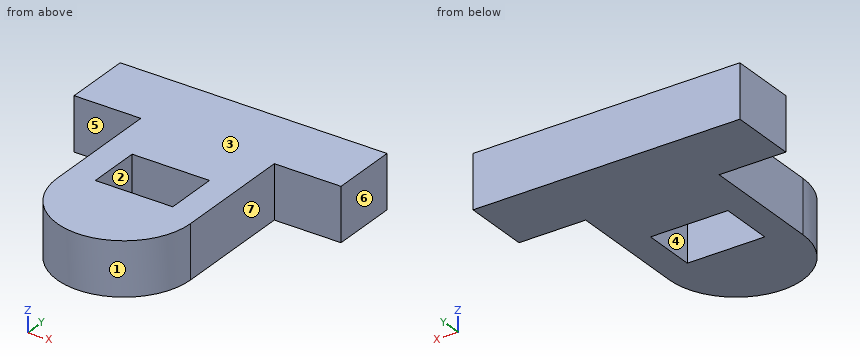
from build123d import *

# Parameters (mm, degrees)
BOSS_EXTRUDE1_DEPTH = 5.08
CUT_EXTRUDE1_DEPTH  = 32.75406374


with BuildPart() as part:
    # Sketch1 → Boss-Extrude1 (new body)
    with BuildSketch(Plane.XY):
        with BuildLine():
            Line((12.7, 18.542), (19.05, 18.542))
            Line((19.05, 18.542), (19.05, 24.892))
            Line((19.05, 24.892), (-6.35, 24.892))
            Line((-6.35, 24.892), (-6.35, 18.542))
            Line((-6.35, 18.542), (0, 18.542))
            Line((0, 18.542), (0, 6.985))
            ThreePointArc((0, 6.985), (6.35, 0.635), (12.7, 6.985))
            Line((12.7, 6.985), (12.7, 18.542))
        make_face()
    extrude(amount=BOSS_EXTRUDE1_DEPTH)

    # Sketch2 → Cut-Extrude1 (cut, through all)
    with BuildSketch(Plane.XY.offset(5.08)):
        Polygon((6.35, 13.462), (10.033, 13.462), (10.033, 8.382), (2.667, 8.382), (2.667, 13.462), align=None)
    extrude(amount=-CUT_EXTRUDE1_DEPTH, mode=Mode.SUBTRACT)


solid = part.part
Geometry: final body of the model. Coordinates: model frame, mm. Face numbers are marked on the shaded views. A direction names the side the tool comes from. Coordinates: 2 decimals unless noted, no trailing zeros. Order: outer loops, then holes, each group sorted by start corner. A loop starts at its lowest first (then second) coordinate and runs counter-clockwise, first axis right, second up. Notation, with made-up numbers: M -18,20 L -4,20 A24 ccw -4,38 Z; hole C -23.75,-29 d2. An arc over 180 degrees is marked long. One line per question, with ' | ' between items. Start each with the question number.
Item 1: Cut plane A-A, the plane x = 6.35. Return the cut outline in (y, z) (3 decimals).
Item 2: Cut plane D-D, the plane y = 16.75. Return the cut outline in (x, z), then the cut area to 3 significant figures.
Item 3: Ray query, probe 1 along X at (y, z) = (12, 4.8); probe 2 along X at (y, z) = (8, 0.3); probe 3 along Y at (x, z) = (15.25, 0.5). Return the intervals inside material, ascending. Write a range as [from, to].
Item 4: Draft query along Y for the marked faces 1, 2 and 3. Return one class per face: released by +Y, released by -Y, zero draft, split by the parting line, or undercut.
Item 5: Pin query (flat end, axial travel): pin 1 Ø2.5 at (y, z) = (12, 1.5) entering from +X; pin 2 Ø2.5 at (x, z) = (16.5, 3.5) entering from -Y; pin 3 Ø1.5 at (x, z) = (8.5, 1) entering from -Y. Return the tip coordinate at first contact, or that it passes through.
Item 6: Cut plane B-B, the plane z = 2. Return the cut outline in (x, y) (3 decimals).
Item 7: Cut plane C-C, the plane x = -1.25. Return the cut outline in (y, z), then the cut area to 3 significant figures.
Item 8: Set-up query: the marked faces 4, 5, 6 and 7. Return all of +Z, -Z, +X, -X, +Y, -Y with unobstructed straight access to the full face (end or side cutting, diameter ignored); none if empty.
A:
1) outline: M 0.635,0 L 8.382,0 L 8.382,5.08 L 0.635,5.08 Z; M 13.462,0 L 24.892,0 L 24.892,5.08 L 13.462,5.08 Z
2) outline: M 0,0 L 12.7,0 L 12.7,5.08 L 0,5.08 Z | area: 64.5 mm2
3) probe 1: x = [0, 2.67], [10.03, 12.7] | probe 2: x = [0, 12.7] | probe 3: y = [18.54, 24.89]
4) face 1: released by -Y | face 2: undercut | face 3: zero draft
5) pin 1: stops at x = 12.7 | pin 2: stops at y = 18.54 | pin 3: stops at y = 0.79
6) outline: M -6.35,18.542 L 0,18.542 L 0,6.985 A6.35 ccw 12.7,6.985 L 12.7,18.542 L 19.05,18.542 L 19.05,24.892 L -6.35,24.892 Z; hole M 2.667,8.382 L 10.033,8.382 L 10.033,13.462 L 2.667,13.462 Z
7) outline: M 18.54,0 L 24.89,0 L 24.89,5.08 L 18.54,5.08 Z | area: 32.3 mm2
8) face 4: +Z, -Z | face 5: +Z, -Z, -X, -Y | face 6: +Z, -Z, +X, +Y, -Y | face 7: +Z, -Z, +X, -Y
